Part print with two shaded views. Sizes in mm from the minimum x, y, z corner. Give positions to 0.01 mm unless a question says otherwise; leave off trailing zeros. Order: outer loops, then holes, each group sorted by start corner. A loop starts at its lowest first (then second) coordinate and runs counter-clockwise, first axis right, second up. Notation, with made-up numbers: M 26.5,-36 L 45.5,-36 A30 ccw 45.5,-6 Z; hole C -10.75,13.25 d3. An arc over 180 degrees is marked long. Return JSON: item names as keys, results as strings. Group by question number.
1. Pin check, flat tips, straight feed: pin 1 (2 mm diameter, centred on x = 91, y = 11.5, fed in from +Z); pin 2 (2 mm diameter, centred on y = 51.5, z = 30, fed in from -X); pin 3 (3 mm diameter, centred on y = 38.5, z = 67, fed in from +X); pin 4 (10 mm diameter, centred on x = 22.5, z = 58, fed in from +Y). Stop position of each tip, or through.
2. Wall check: probe 1 along X at (y, z) = (61, 53.5); probe 2 along Z at (x, y) = (72.5, 60.5). Give the ranges that are in metal, low to high. Write a range as [from, to].
3. Slice it at C-C on y = 9. List the corners of the cut face in (x, z), then the cut area to 3 significant figures.
4. Two-plate mould, pull along Z, no slides. Class the marked faces 1, 2 and 3: released by +Z, released by -Z, zero draft, split by the parting line, or undercut.
5. Slice it at B-B on z = 53.5. List the corners of the cut face in (x, y).
6. Slice it at A-A on x = 53.5. List the corners of the cut face in (y, z).
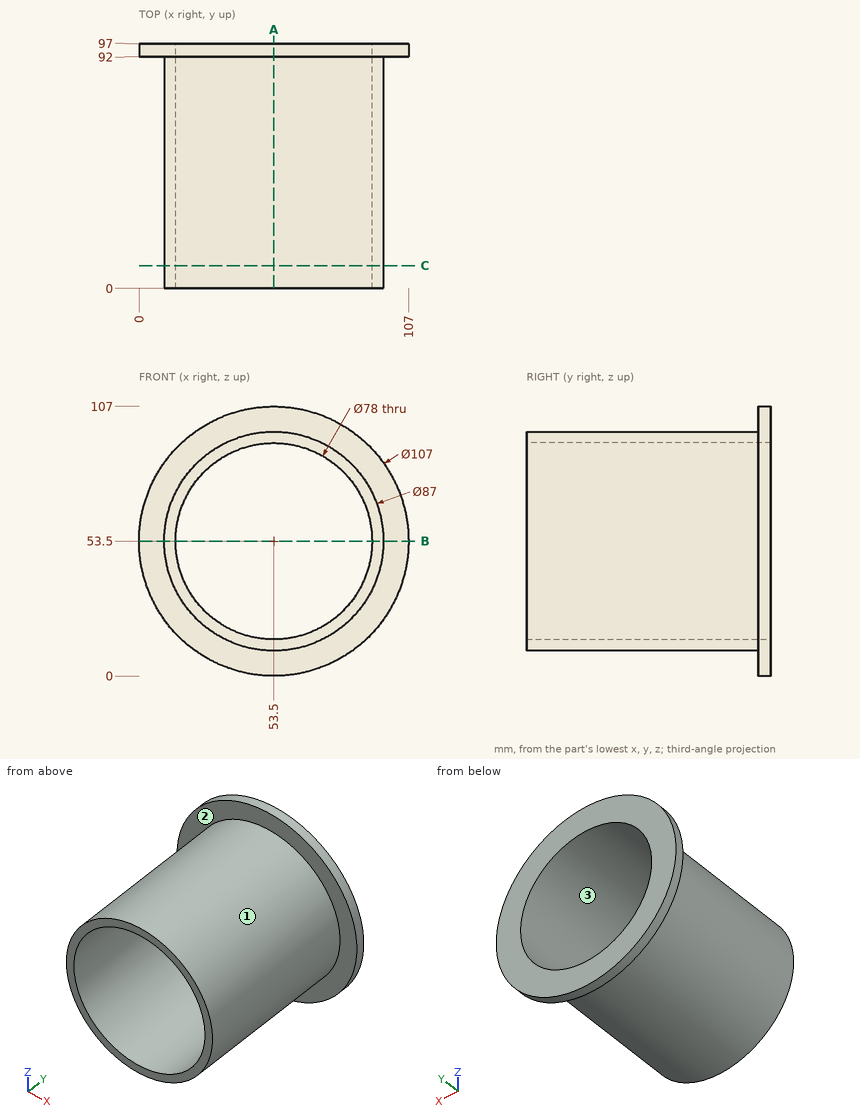
Result:
{
 "1": {"pin 1": "stops at z = 77.16", "pin 2": "stops at x = 16.27", "pin 3": "stops at x = 95.31", "pin 4": "passes through"},
 "2": {"probe 1": "x = [10, 14.5], [92.5, 97]", "probe 2": "z = [14.37, 19.44], [87.56, 92.63]"},
 "3": {"outline": "C 53.5,53.5 d87; hole C 53.5,53.5 d78", "area": "1,170 mm2"},
 "4": {"face 1": "split by the parting line", "face 2": "zero draft", "face 3": "undercut"},
 "5": {"outline": "M 0,92 L 10,92 L 10,0 L 14.5,0 L 14.5,97 L 0,97 Z; M 92.5,0 L 97,0 L 97,92 L 107,92 L 107,97 L 92.5,97 Z"},
 "6": {"outline": "M 0,10 L 92,10 L 92,0 L 97,0 L 97,14.5 L 0,14.5 Z; M 0,92.5 L 97,92.5 L 97,107 L 92,107 L 92,97 L 0,97 Z"}
}
